Could you check a few things on this model? Use its own coordinates, in mm. Face numbers are marked on the shaded views. A direction names the side the tool comes from. Round coordinates to 2 decimals unless told otherwise and drop trailing zeros. Order: outer loops, then holes, each group sorted by start corner. A loop starts at its lowest first (then second) coordinate and runs counter-clockwise, first axis right, second up. Notation, with made-up numbers: (68, -39.5) -> (77, -39.5) arc R23 ccw to (77, -9.5) -> close; hole circle Ø4 at (51, 84.5). An arc over 180 degrees is marked (long way). One line per question, with ' | ' between items.
```python
from build123d import *

# Parameters (mm, degrees)
SKETCH1_R           = 25
BOSS_EXTRUDE1_DEPTH = 4
SKETCH2_R           = 4
BOSS_EXTRUDE2_DEPTH = 8


with BuildPart() as part:
    # Sketch1 → Boss-Extrude1 (new body)
    with BuildSketch(Plane(origin=(0, 0, 0), x_dir=(1, 0, 0), z_dir=(0, 1, 0))):
        with Locations(Location((0, 0, 0), (0, 0, 270))):
            Circle(SKETCH1_R)
    extrude(amount=BOSS_EXTRUDE1_DEPTH)

    # Sketch2 → Boss-Extrude2 (add)
    with BuildSketch(Plane.XZ):
        with Locations(Location((0, 0, 0), (0, 0, 270))):
            Circle(SKETCH2_R)
        with BuildLine():
            Line((-2.258317958, 0.95), (-0.95, 0.95))
            Line((-0.95, 0.95), (-0.95, 2.258317958))
            ThreePointArc((-0.95, 2.258317958), (0, 2.45), (0.95, 2.258317958))
            Line((0.95, 2.258317958), (0.95, 0.95))
            Line((0.95, 0.95), (2.258317958, 0.95))
            ThreePointArc((2.258317958, 0.95), (2.45, 0), (2.258317958, -0.95))
            Line((2.258317958, -0.95), (0.95, -0.95))
            Line((0.95, -0.95), (0.95, -2.258317958))
            ThreePointArc((0.95, -2.258317958), (0, -2.45), (-0.95, -2.258317958))
            Line((-0.95, -2.258317958), (-0.95, -0.95))
            Line((-0.95, -0.95), (-2.258317958, -0.95))
            ThreePointArc((-2.258317958, -0.95), (-2.45, 0), (-2.258317958, 0.95))
        make_face(mode=Mode.SUBTRACT)
    extrude(amount=BOSS_EXTRUDE2_DEPTH)


solid = part.part
```
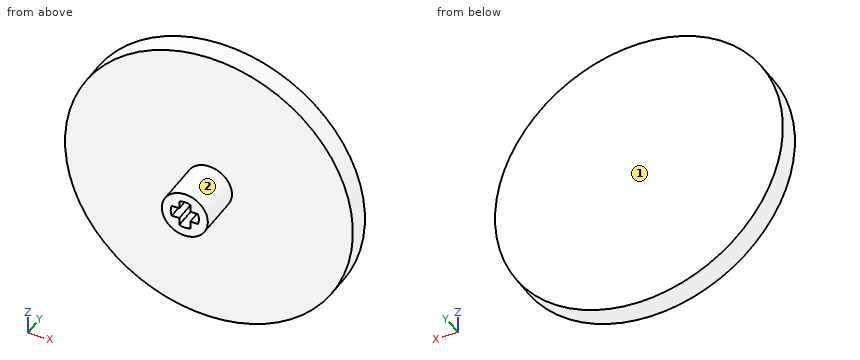
1. I want a section at B-B on z = 0. List the corners of the cut face in (x, y) for me, and give its area (3 significant figures).
From the geometry:
outline: (-25, 0) -> (-4, 0) -> (-4, -8) -> (-2.45, -8) -> (-2.45, 0) -> (2.45, 0) -> (2.45, -8) -> (4, -8) -> (4, 0) -> (25, 0) -> (25, 4) -> (-25, 4) -> close | area: 225 mm²
2. I'm going to push flat-ended pins straight in: pin 1 (1 mm diameter, centred on y = -4.5, z = 1.5, fed in from +X); pin 2 (1.5 mm diameter, centred on y = -3, z = -0.5, fed in from +X); pin 3 (0.7 mm diameter, centred on y = -3, z = 2, fed in from -X). Where does each tip first touch, or does it pass through?
From the geometry:
pin 1: stops at x = 3.87 | pin 2: stops at x = 4 | pin 3: stops at x = -3.64
3. I want a section at D-D on y = 3. List the corners of the cut face in (x, z) for me, and give its area (3 significant figures).
From the geometry:
outline: circle Ø50 at (0, 0) | area: 1,960 mm²
4. I need wall thicknesses on probe 1 along Y at (x, z) = (21, 13); probe 2 along X at (y, z) = (-2, -1); probe 3 along Z at (x, y) = (2, -1.75). Which ranges of each line are inside material? Lowest first, please.
From the geometry:
probe 1: y = 0 to 4 | probe 2: x = -3.87 to -0.95, 0.95 to 3.87 | probe 3: z = -3.46 to -0.95, 0.95 to 3.46
5. I want a section at A-A on y = -2.25. List the corners of the cut face in (x, z) for me.
From the geometry:
outline: circle Ø8 at (0, 0); hole (-2.26, -0.95) -> (-0.95, -0.95) -> (-0.95, -2.26) arc R2.45 ccw to (0.95, -2.26) -> (0.95, -0.95) -> (2.26, -0.95) arc R2.45 ccw to (2.26, 0.95) -> (0.95, 0.95) -> (0.95, 2.26) arc R2.45 ccw to (-0.95, 2.26) -> (-0.95, 0.95) -> (-2.26, 0.95) arc R2.45 ccw to start
6. I want a section at C-C on x = 0. List the corners of the cut face in (y, z) for me.
From the geometry:
outline: (-8, -4) -> (0, -4) -> (0, -25) -> (4, -25) -> (4, 25) -> (0, 25) -> (0, 4) -> (-8, 4) -> (-8, 2.45) -> (0, 2.45) -> (0, -2.45) -> (-8, -2.45) -> close
7. On a 3-axis mill with a long thin cutter (end or side, diameter ignored), from which of +Z, -Z, +X, -X, +Y, -Y can I reach the whole of each face in a straight line? I mean the marked faces 1 and 2. Say none if no direction works.
From the geometry:
face 1: +Z, -Z, +X, -X, +Y | face 2: -Y
